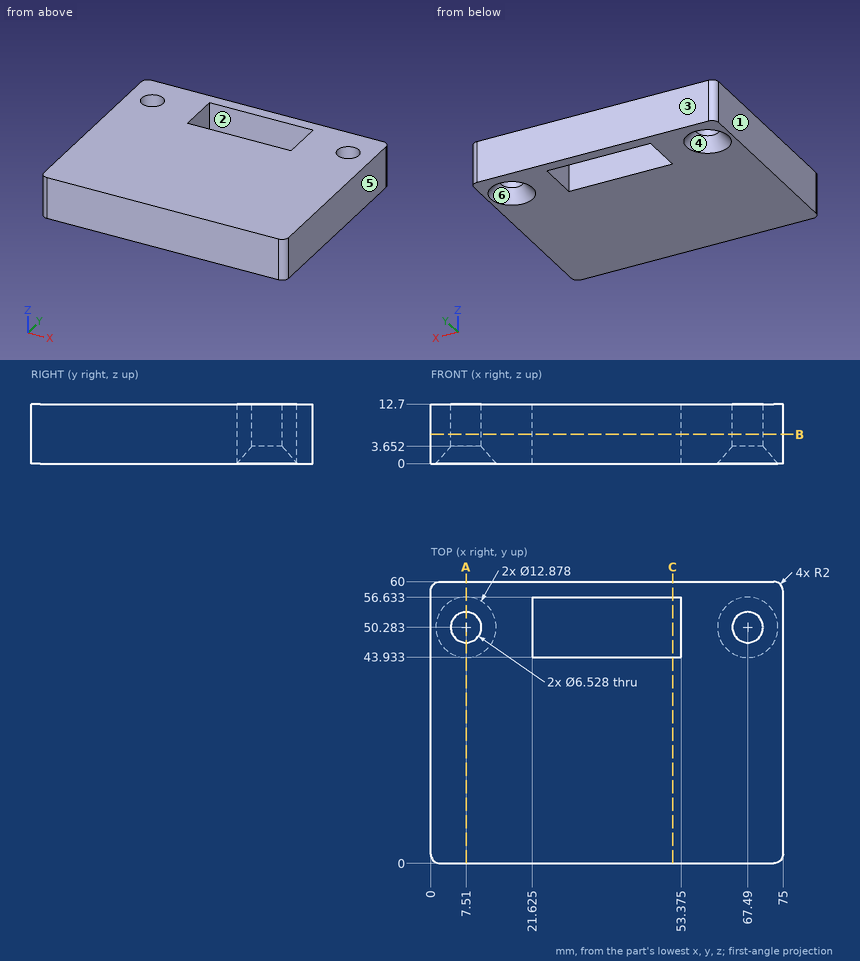
Design review of the part shown in the three views and the two pictorial views. Dimensions are in mm from the part's minimum x, y and z. A direction names the side the tool comes from. Round coordinates to 2 decimals unless told otherwise and drop trailing zeros. Write each loop counter-clockwise with the first axis right and the second up, starting at its lowest first coordinate (ties: lowest second). Pieces come first, ordered by that corner, then holes. Notation, with made-up numbers: (-32, 83) - (15, 83) arc R25 ccw to (15, 118) - close; hole circle Ø11 at (-30.75, 7.25). An arc over 180 degrees is marked (long way). Write item = value, one per line. Start each with the question number.
1. For the marked faces 1 and 2, list the 3-axis set-ups (+Z, -Z, +X, -X, +Y, -Y) from which the entire face can be reached by the end or side of a thin tool; tool diameter is ignored.
2. Wall thickness on L1, parallel to Y at x = 7.51, z = 6; L2, parallel to X at y = 46, z = 7 (1 decimal); L3, parallel to Y at x = 28, z = 8.75: over which ranges is each line inside the solid? List them lowest first.
3. Consider section A-A on x = 7.51. State the section outline as (y, z) points.
4. Draft analysis for pull direction X (two halves, no side actions). For the marked faces 3, 4, 5 and 6, state which applies: released by +X, released by -X, zero draft, split by the parting line, or undercut.
5. Consider section B-B on z = 6.25. State the section outline as (x, y) points (1 decimal), plus the area to 3 significant figures.
6. For pin 1 Ø5 at (x, z) = (65, 11) entering from -Y, flat-tipped, find the tip position at first contact; note if it passes through.
7. Consider section C-C on x = 51.5. State the section outline as (y, z) points, plus the area to 3 significant figures.
Evaluation:
q1.face_1 = +Z, -Z, -X, +Y, -Y
q1.face_2 = +Z, -Z
q2.L1 = 0 to 47.02, 53.55 to 60
q2.L2 = 0 to 21.6, 53.4 to 75
q2.L3 = 0 to 43.93, 56.63 to 60
q3.outline = (0, 0) - (43.84, 0) - (47.02, 3.65) - (47.02, 12.7) - (0, 12.7) - close; (53.55, 3.65) - (56.72, 0) - (60, 0) - (60, 12.7) - (53.55, 12.7) - close
q4.face_3 = zero draft
q4.face_4 = undercut
q4.face_5 = released by +X
q4.face_6 = undercut
q5.outline = (0, 2) arc R2 ccw to (2, 0) - (73, 0) arc R2 ccw to (75, 2) - (75, 58) arc R2 ccw to (73, 60) - (2, 60) arc R2 ccw to (0, 58) - close; hole circle Ø6.5 at (7.5, 50.3); hole (21.6, 43.9) - (53.4, 43.9) - (53.4, 56.6) - (21.6, 56.6) - close; hole circle Ø6.5 at (67.5, 50.3)
q5.area = 4,030 mm2
q6.pin_1 = 0
q7.outline = (0, 0) - (43.93, 0) - (43.93, 12.7) - (0, 12.7) - close; (56.63, 0) - (60, 0) - (60, 12.7) - (56.63, 12.7) - close
q7.area = 601 mm2
